The model under review builds one solid part; all positions refer to its coordinate system, in mm. A direction names the side the tool comes from. Give positions to 0.01 mm unless a question says otherwise; leave off trailing zeros. Order: outer loops, then holes, each group sorted by start corner. A loop starts at its lowest first (then second) coordinate and runs counter-clockwise, first axis right, second up. Notation, with made-up numbers: (49, 15) - (69, 15) arc R16 cw to (69, 21) - close; hole circle Ø9 at (-6, 20.5). An arc over 180 degrees is marked (long way). Use a Markdown table: item, result. Add a question column.
```python
from build123d import *
from OCP.BRepFilletAPI import BRepFilletAPI_MakeFillet

# Parameters (mm, degrees)
ESQUISSE1_R             = 1.2
BOSS_EXTRU_1_DEPTH      = 6.4
BOSS_EXTRU_2_START      = -3.2
ESQUISSE4_W             = 0.6
ESQUISSE4_H             = 3.5
BOSS_EXTRU_2_DEPTH      = 1.6
ESQUISSE5_R             = 0.8
ENL_V_MAT_EXTRU_1_DEPTH = 23.054081255
ESQUISSE6_W             = 1
ESQUISSE6_H             = 4.4
ENL_V_MAT_EXTRU_2_DEPTH = 1.6
ESQUISSE6_3_W           = 2
ESQUISSE6_3_H           = 3.55
BOSS_EXTRU_3_DEPTH      = 1.2
CONG_2_R                = 1
CONG_2_R_2              = 0.5
ESQUISSE7_R             = 1
BOSS_EXTRU_9_DEPTH      = 0.1
BOSS_EXTRU_10_START     = -6.5
ESQUISSE7_3_R           = 1
BOSS_EXTRU_10_DEPTH     = 0.1
CONG_1_R                = 0.4


with BuildPart() as part:
    # Esquisse1 → Boss.-Extru.1 (new body)
    with BuildSketch(Plane.XY):
        Polygon((0, 0), (19.8, 0), (19.8, 9.9), (10.65, 9.9), (9.95, 10.6), (0, 10.6), align=None)
        with Locations((5.1, 2.5)):
            Circle(ESQUISSE1_R, mode=Mode.SUBTRACT)
        with Locations((13.6, 2.5)):
            Circle(ESQUISSE1_R, mode=Mode.SUBTRACT)
    extrude(amount=BOSS_EXTRU_1_DEPTH)

    # Esquisse4 → Boss.-Extru.2 (add, symmetric)
    with BuildSketch(Plane.XY.offset(6.4).offset(BOSS_EXTRU_2_START)):
        with Locations((17.95, -1.75)):
            Rectangle(ESQUISSE4_W, ESQUISSE4_H)
        with Locations((10.65, -1.75)):
            Rectangle(ESQUISSE4_W, ESQUISSE4_H)
        with Locations((1.85, -1.75)):
            Rectangle(ESQUISSE4_W, ESQUISSE4_H)
    extrude(amount=BOSS_EXTRU_2_DEPTH, both=True)

    # Esquisse5 → Enlèv. mat.-Extru.1 (cut, through all)
    with BuildSketch(Plane(origin=(18.25, 0, 0), x_dir=(0, 0, -1), z_dir=(1, 0, 0))):
        with Locations(Location((-3.111189777, -1.9, 0), (0, 0, 90))):
            Circle(ESQUISSE5_R)
    extrude(amount=-ENL_V_MAT_EXTRU_1_DEPTH, mode=Mode.SUBTRACT)

    # Esquisse6 → Enlèv. mat.-Extru.2 (cut)
    with BuildSketch(Plane(origin=(0, 10.6, 0), x_dir=(1, 0, 0), z_dir=(0, 1, 0))):
        with Locations((3.7, -3.2)):
            Rectangle(ESQUISSE6_W, ESQUISSE6_H)
    extrude(amount=-ENL_V_MAT_EXTRU_2_DEPTH, mode=Mode.SUBTRACT)

    # Esquisse6<3> → Boss.-Extru.3 (add)
    with BuildSketch(Plane(origin=(0, 10.6, 0), x_dir=(1, 0, 0), z_dir=(0, 1, 0))):
        with Locations((7.1, -2.975)):
            Rectangle(ESQUISSE6_3_W, ESQUISSE6_3_H)
    extrude(amount=BOSS_EXTRU_3_DEPTH)

    # Congé2
    cong_2_edges_1 = [part.edges().sort_by_distance(p)[0] for p in [
        (8.1, 11.8, 2.975),
        (6.1, 11.8, 2.975),
    ]]
    cong_2_edges_2 = [part.edges().sort_by_distance(p)[0] for p in [
        (7.1, 11.8, 4.75),
        (7.1, 11.8, 1.2),
    ]]
    cong_2 = BRepFilletAPI_MakeFillet(part.part.solid().wrapped)
    for e in cong_2_edges_1:
        cong_2.Add(CONG_2_R - 0.0001, e.wrapped)
    for e in cong_2_edges_2:
        cong_2.Add(CONG_2_R_2 - 0.0001, e.wrapped)
    add(Compound.cast(cong_2.Shape()), mode=Mode.REPLACE)  # a hair under: the kernel refuses the full size

    # Esquisse7 → Boss.-Extru.9 (add)
    with BuildSketch(Plane(origin=(0, 0, 0), x_dir=(-1, 0, 0), z_dir=(0, 0, -1))):
        with Locations(Location((-3.2, 9.1, 0), (0, 0, 180))):
            Circle(ESQUISSE7_R)
    extrude(amount=BOSS_EXTRU_9_DEPTH)

    # Esquisse7<3> → Boss.-Extru.10 (add)
    with BuildSketch(Plane(origin=(0, 0, 0), x_dir=(-1, 0, 0), z_dir=(0, 0, -1)).offset(BOSS_EXTRU_10_START)):
        with Locations(Location((-3.2, 9.1, 0), (0, 0, 180))):
            Circle(ESQUISSE7_3_R)
    extrude(amount=BOSS_EXTRU_10_DEPTH)

    # Congé1
    cong_1_edges = [part.edges().sort_by_distance(p)[0] for p in [
        (0, 10.6, 3.2),
        (19.8, 9.9, 3.2),
        (19.8, 0, 3.2),
        (0, 0, 3.2),
        (17.95, -3.5, 1.6),
        (17.95, -3.5, 4.8),
        (10.65, -3.5, 1.6),
        (10.65, -3.5, 4.8),
        (1.85, -3.5, 1.6),
        (1.85, -3.5, 4.8),
    ]]
    fillet(cong_1_edges, radius=CONG_1_R)


solid = part.part
```
Q1. We need section C-C (z = 0.75). Write out the cut boundary in (x, y), plus the area to 3 significant figures.
Q2. Wall thickness on probe 1 along Z at (x, y) = (10.5, -1.9); probe 2 along Y at (x, z) = (5.1, 3.5); probe 3 along X at (y, z) = (1.75, 5.25): over which ranges is each line inside the solid? List them lowest first.
Q3. We need section D-D (y = -1.9). Write out the cut boundary in (x, z).
Q4. Clearance check with flat-ended pins moving along their axes: P1, Ø2.5, axis at y = -1, z = 2.5, coming from the -X side; P2, Ø1, axis at y = -1.5, z = 4, coming from the -X side; P3, Ø3, axis at x = 5.1, y = 2.5, coming from the +Z side. State where each tip first meets the part, or that it passes through.
Q5. We need section A-A (x = 13.6). Write out the cut boundary in (y, z).
Q6. Machinability: for faces 1 (the flat face through (4, 10, 5.4)), 2 (the flat face through (19.8, 5, 3)), 3 (the cylindrical face through (17.954, -1.47, 3.786)), 4 (the flat face through (15, 9.9, 3)), 5 (the flat face through (10.35, -1, 4)), which of the approach directions +Z, -Z, +X, -X, +Y, -Y give a long, thin tool a straight path to every point of the face, cutting with its end or side? Answer none if there is none.
Q7. We need section B-B (y = 2.5). Write out the cut boundary in (x, z).
Q8. Draft analysis for pull direction Y (two halves, no side actions). For faces 6 (the cylindrical face through (14.25, 3.51, 3.16)), 7 (the flat face through (4, 9, 3)), 8 (the flat face through (10.95, -1, 4)), state which applies: pulls with the +Y half, pulls with the -Y half, needs draft (parallel to the pull), parting line crosses it, or undercut.
Here are the results:
| question | item | result |
|---|---|---|
| 1 | outline | (0, 0.4) arc R0.4 ccw to (0.4, 0) - (19.4, 0) arc R0.4 ccw to (19.8, 0.4) - (19.8, 9.5) arc R0.4 ccw to (19.4, 9.9) - (10.65, 9.9) - (9.95, 10.6) - (0.4, 10.6) arc R0.4 ccw to (0, 10.2) - close; hole circle Ø2.4 at (5.1, 2.5); hole circle Ø2.4 at (13.6, 2.5) |
| 1 | area | 194 mm2 |
| 2 | probe 1 | 1.6 to 2.31, 3.91 to 4.8 |
| 2 | probe 2 | 0 to 1.3, 3.7 to 10.6 |
| 2 | probe 3 | 0 to 4.16, 6.04 to 12.66, 14.54 to 19.8 |
| 3 | outline | (1.55, 1.6) - (2.15, 1.6) - (2.15, 2.31) - (1.55, 2.31) - close; (1.55, 3.91) - (2.15, 3.91) - (2.15, 4.8) - (1.55, 4.8) - close; (10.35, 1.6) - (10.95, 1.6) - (10.95, 2.31) - (10.35, 2.31) - close; (10.35, 3.91) - (10.95, 3.91) - (10.95, 4.8) - (10.35, 4.8) - close; (17.65, 1.6) - (18.25, 1.6) - (18.25, 2.31) - (17.65, 2.31) - close; (17.65, 3.91) - (18.25, 3.91) - (18.25, 4.8) - (17.65, 4.8) - close |
| 4 | P1 | x = 0.03 |
| 4 | P2 | x = 1.55 |
| 4 | P3 | z = 6.4 |
| 5 | outline | (0, 0) - (1.3, 0) - (1.3, 6.4) - (0, 6.4) - close; (3.7, 0) - (9.9, 0) - (9.9, 6.4) - (3.7, 6.4) - close |
| 6 | face 1 | +Y |
| 6 | face 2 | +Z, -Z, +X, +Y, -Y |
| 6 | face 3 | +X, -X |
| 6 | face 4 | +Z, -Z, +X, +Y |
| 6 | face 5 | +Z, -Z, -Y |
| 7 | outline | (0, 0) - (3.9, 0) - (3.9, 6.4) - (0, 6.4) - close; (6.3, 0) - (12.4, 0) - (12.4, 6.4) - (6.3, 6.4) - close; (14.8, 0) - (19.8, 0) - (19.8, 6.4) - (14.8, 6.4) - close |
| 8 | face 6 | undercut |
| 8 | face 7 | pulls with the +Y half |
| 8 | face 8 | needs draft |
